Input: dimensioned drawing with shaded views. Units: mm. Origin: part minimum x, y, z. A direction names the side the tool comes from. Coordinates: 2 decimals unless noted, no trailing zeros. Order: outer loops, then holes, each group sorted by start corner. A loop starts at its lowest first (then second) coordinate and runs counter-clockwise, first axis right, second up. Notation, with made-up numbers: (56.5, -2.5) - (114.5, -2.5) arc R32 cw to (114.5, 36.5) - close; hole circle Ø8 at (-6, 35.5). An arc over 180 degrees is marked (long way). Use one line per item in the form item = value. Start each with the question number.
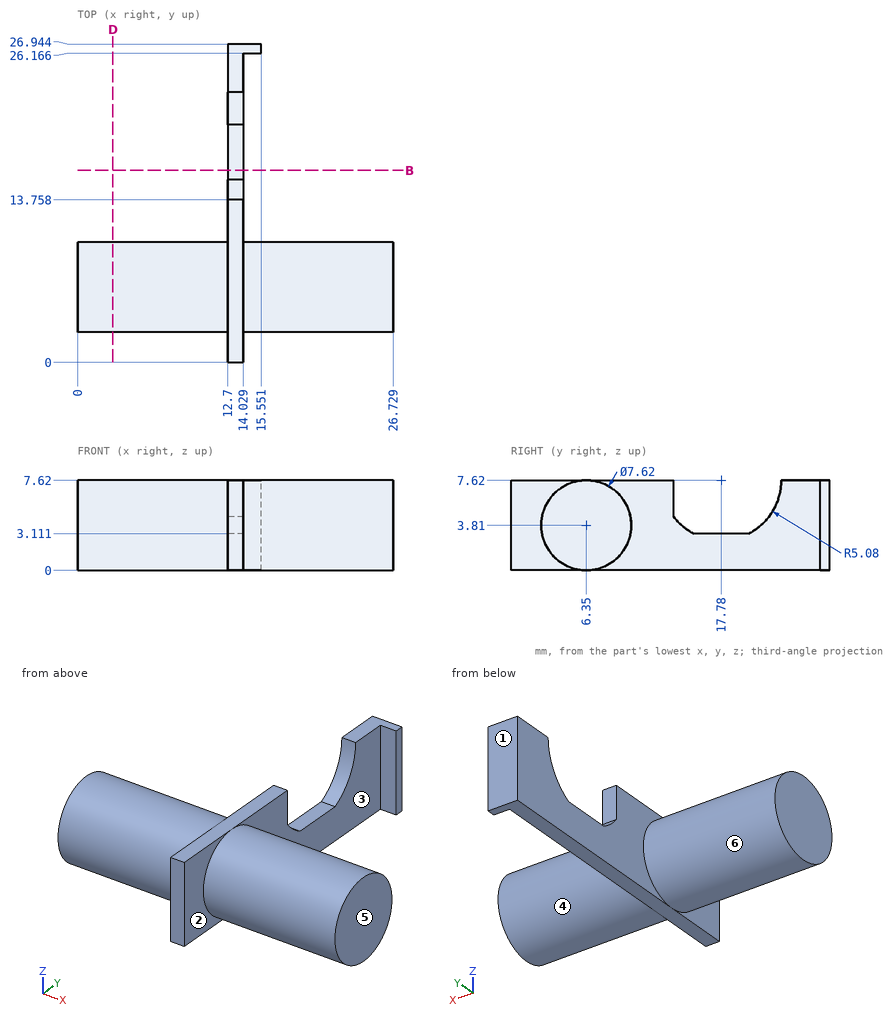
(1) Set-up query: the marked faces 4, 5 and 6. Return all of +Z, -Z, +X, -X, +Y, -Y with unobstructed straight access to the full face (end or side cutting, diameter ignored); none if empty.
(2) Material intervals for L1, parallel to X at y = 16.5, z = 2; L2, parallel to Y at x = 21.25, z = 4.5; L3, parallel to Z at x = 19.25, y = 5.25, sorted ascending. Write a range as from..to.
(3) Contact query for flat-ended pins moving along their axis: pin 1 Ø1.9 at (y, z) = (1.5, 3) entering from -X; pin 2 Ø0.9 at (y, z) = (26.5, 5.5) entering from +X; pin 3 Ø1 at (x, z) = (2.5, 1.5) entering from -Y. Output: stop coordinate, or through.
(4) Cut plane D-D on x = 3. Return the cut outline in (y, z), plus the area to 3 significant figures.
(5) Draft query along Y for the marked faces 1, 2 and 3. Return one class per face: released by +Y, released by -Y, zero draft, split by the parting line, or undercut.
(6) Cut plane B-B on y = 16.25. Return the cut outline in (x, z).
Check sheet entries:
q1.face_4 = +X
q1.face_5 = +Z, -Z, +X, +Y, -Y
q1.face_6 = -X
q2.L1 = 12.7..14.03
q2.L2 = 2.6..10.1
q2.L3 = 0.16..7.46
q3.pin_1 = 12.7
q3.pin_2 = 15.55
q3.pin_3 = 3
q4.outline = circle Ø7.62 at (6.35, 3.81)
q4.area = 45.6 mm^2
q5.face_1 = released by +Y
q5.face_2 = zero draft
q5.face_3 = undercut
q6.outline = (12.7, 0) - (14.03, 0) - (14.03, 3.11) - (12.7, 3.11) - close
